```python
from build123d import *

# Parameters (mm, degrees)
EXTRUDE1_DEPTH     = 2.36
SKETCH2_R          = 5
EXTRUDE2_DEPTH     = 13.52
SKETCH3_R          = 4.5
CUT_EXTRUDE1_DEPTH = 13.52
SKETCH4_R          = 0.5
EXTRUDE3_DEPTH     = 6.5
SKETCH5_R          = 0.5
EXTRUDE4_DEPTH     = 9


with BuildPart() as part:
    # Sketch1 → Extrude1 (new body)
    with BuildSketch(Plane.XY):
        with BuildLine():
            Line((1, 0), (16.45, 0))
            ThreePointArc((16.45, 0), (17.157106781, -0.292893219), (17.45, -1))
            Line((17.45, -1), (17.45, -16.45))
            ThreePointArc((17.45, -16.45), (17.157106781, -17.157106781), (16.45, -17.45))
            Line((16.45, -17.45), (1, -17.45))
            ThreePointArc((1, -17.45), (0.292893219, -17.157106781), (0, -16.45))
            Line((0, -16.45), (0, -1))
            ThreePointArc((0, -1), (0.292893219, -0.292893219), (1, 0))
        make_face()
    extrude(amount=EXTRUDE1_DEPTH)

    # Sketch2 → Extrude2 (add)
    with BuildSketch(Plane(origin=(0, 0, 0), x_dir=(-1, 0, 0), z_dir=(0, 0, -1))):
        with Locations((-8.725, -8.725)):
            Circle(SKETCH2_R)
    extrude(amount=EXTRUDE2_DEPTH)

    # Sketch3 → Cut-Extrude1 (cut)
    with BuildSketch(Plane(origin=(0, 0, -13.52), x_dir=(-1, 0, 0), z_dir=(0, 0, -1))):
        with Locations((-8.725, -8.725)):
            Circle(SKETCH3_R)
    extrude(amount=-CUT_EXTRUDE1_DEPTH, mode=Mode.SUBTRACT)

    # Sketch4 → Extrude3 (add)
    with BuildSketch(Plane.XY.offset(2.36)):
        with Locations((8.725, -8.725)):
            Circle(SKETCH4_R)
        with Locations((15.075, -2.375)):
            Circle(SKETCH4_R)
        with Locations((2.375, -2.375)):
            Circle(SKETCH4_R)
        with Locations((2.375, -15.075)):
            Circle(SKETCH4_R)
        with Locations((15.075, -15.075)):
            Circle(SKETCH4_R)
    extrude(amount=EXTRUDE3_DEPTH)

    # Sketch5 → Extrude4 (add)
    with BuildSketch(Plane(origin=(0, 0, 0), x_dir=(-1, 0, 0), z_dir=(0, 0, -1))):
        with Locations((-8.725, -8.725)):
            Circle(SKETCH5_R)
    extrude(amount=EXTRUDE4_DEPTH)


solid = part.part
```
Source: CAD feature listing. Evaluate the final solid. Frame: model axes, mm. A direction names the side the tool comes from. Give positions to 0.01 mm unless a question says otherwise; leave off trailing zeros. Loops run counter-clockwise (first coordinate to the right, second up) from the corner with the lowest first, then second, coordinate; pieces in that order, holes last. Notation, with made-up numbers: (74.25, 34.25) -> (103.25, 34.25) arc R16 cw to (103.25, 55.25) -> close; hole circle Ø5 at (80, 24). An arc over 180 degrees is marked (long way). Put each result on its own line as item: value. Start each with the question number.
1) Cut plane A-A (x = 15). Return loops of the section in (y, z), then the cut area to 3 significant figures.
2) Draft query along Y for faces 1 (the face through (2.4, -2.4, 8.86)), 2 (the face through (15.537, -15.267, 5.564)), 3 (the face through (9.094, -8.387, -4.437)), 4 (the face through (0.301, -17.165, 1.163)). Return one class per face: released by +Y, released by -Y, zero draft, split by the parting line, or undercut.
3) Material intervals for probe 1 along Z at (x, y) = (1.5, -13.5); probe 2 along Y at (x, z) = (9, -11.25); probe 3 along Y at (x, z) = (12.75, -2.5), sorted ascending.
4) Reachability of faces 5 (the face through (8.7, -8.7, -9)), 6 (the face through (8.7, -8.7, 8.86)), 7 (the face through (8.225, -8.703, 5.564)) from +Z, -Z, +X, -X, +Y, -Y: full face, straight path, thin tool, end or side. Return the list, or none.
5) Contact query for flat-ended pins moving along their axis: P1, Ø3, axis at x = 5.5, y = -12.5, coming from the +Z side; P2, Ø0.5, axis at x = 8.5, y = -9, coming from the -Z side; P3, Ø1, axis at y = -5, z = -6, coming from the -X side. Output: stop coordinate, or through.
6) Cut plane D-D (z = -3.75). Return loops of the section in (x, y) (3 decimals).
7) Cut plane B-B (z = 3.25). Return loops of the section in (x, y) (3 decimals).
8) Cut plane C-C (y = -7.75). Return loops of the section in (x, z), then the cut area to 3 significant figures.
Results are:
1. outline: (-17.45, 0) -> (0, 0) -> (0, 2.36) -> (-1.88, 2.36) -> (-1.88, 8.86) -> (-2.87, 8.86) -> (-2.87, 2.36) -> (-14.58, 2.36) -> (-14.58, 8.86) -> (-15.57, 8.86) -> (-15.57, 2.36) -> (-17.45, 2.36) -> close
1. area: 54.0 mm2
2. face 1: zero draft
2. face 2: undercut
2. face 3: undercut
2. face 4: released by -Y
3. probe 1: z = 0 to 2.36
3. probe 2: y = -13.72 to -13.22, -4.23 to -3.73
3. probe 3: y = -11.69 to -10.74, -6.71 to -5.76
4. face 5: -Z
4. face 6: +Z, +X, -X, +Y, -Y
4. face 7: +Z
5. P1: stops at z = 2.36
5. P2: stops at z = -9
5. P3: stops at x = 4.9
6. outline: circle Ø10 at (8.725, -8.725); circle Ø1 at (8.725, -8.725); hole circle Ø9 at (8.725, -8.725)
7. outline: circle Ø1 at (2.375, -15.075); circle Ø1 at (2.375, -2.375); circle Ø1 at (8.725, -8.725); circle Ø1 at (15.075, -15.075); circle Ø1 at (15.075, -2.375)
8. outline: (0, 0) -> (3.82, 0) -> (3.82, -13.52) -> (4.33, -13.52) -> (4.33, 0) -> (13.12, 0) -> (13.12, -13.52) -> (13.63, -13.52) -> (13.63, 0) -> (17.45, 0) -> (17.45, 2.36) -> (0, 2.36) -> close
8. area: 55.0 mm2
